Can you work these out from the model? Positions are in its coordinate system, mm. A direction names the side the tool comes from. Give positions to 0.01 mm unless a question says otherwise; leave off trailing zeros. Loops run counter-clockwise (first coordinate to the right, second up) from the corner with the lowest first, then second, coordinate; pieces in that order, holes last. Notation, with made-up numbers: (2.5, 20.5) -> (54.5, 20.5) arc R9 ccw to (54.5, 24.5) -> close; hole circle Ø1 at (-33.75, 61.5). An arc over 180 degrees is marked (long way). Return JSON: item names as keys, results as strings. Group by question number.
Q1. Suppose I cut it at C-C, the plane x = -27.75. Please give me the cut outline in (y, z), and give its area (3 significant figures).
Q2. Which directions (+Z, -Z, +X, -X, +Y, -Y) give clear straight access to the entire face, cutting with the end or side of a thin tool? Please do faces 4 (the flat face through (-15, 0, -15)), 5 (the flat face through (-3.5, 1, -21)), 6 (the flat face through (-26.5, 1, -3)).
Q3. Suppose I cut it at A-A, the plane y = 1.05. Please give me the cut outline in (x, z).
Q4. Suppose I cut it at B-B, the plane z = -24.5. Please give me the cut outline in (x, y), and give its area (3 significant figures).
Q5. Will this pin go through, and if not, where does the flat tip stop? pin 1 (12 mm diameter, centred on x = -20, z = -11, fed in from -Y).
Q6. I need wall thicknesses on line 1 along X through (y, z) = (1.3, -20.5); line 2 along Z through (x, y) = (-2.25, 0.75); line 3 along X through (y, z) = (1.2, -11). Which ranges of each line are inside material? Lowest first, please. Write a range as [from, to].
Q7. Thinking about a two-plate mould opening in X: for faces 1 (the flat face through (-26.5, 1, -21)), 2 (the flat face through (-3.5, 1, -3)), 3 (the flat face through (-15, 1.5, -15)), which applies, pulls with the +X half, pulls with the -X half, needs draft (parallel to the pull), parting line crosses it, or undercut?
Autodesk Inventor part; units mm, degrees
ref_plane "YZ Plane" through (0, 0, 0) normal (1, 0, 0) x (0, 1, 0)
ref_plane "XZ Plane" through (0, 0, 0) normal (0, 1, 0) x (-1, 0, 0)
ref_plane "XY Plane" through (0, 0, 0) normal (0, 0, 1) x (1, 0, 0)
sketch "スケッチ1" plane through (0, 0, 0) normal (0, 1, 0) x (-1, 0, 0)
  line L0 (0, 0) -> (30, 0)
  line L1 (30, 0) -> (30, -30)
  line L2 (30, -30) -> (0, -30)
  line L3 (0, -30) -> (0, 0)
  circle A0 centre (26.5, -9) radius 3.5
  circle A1 centre (3.5, -9) radius 3.5
  line L4 (26.5, 0) -> (26.5, -30)
  line L5 (3.5, -30) -> (3.5, 0)
  point P0 (26.5, -12.5)
  point P1 (26.5, -5.5)
  point P2 (3.5, -5.5)
  point P3 (3.5, -12.5)
  dimension "d0" = 30
  dimension "d1" = 30
  dimension "d2" = 7
  dimension "d3" = 7
  dimension "d4" = 9
extrude "押し出し1" add sketch "スケッチ1" along normal blind 1.5 contours L0 L4 A0 L2 L5 A1 | A1 L5 | A1 L5 | L4 A0 | A0 L4
properties part number "type_A"
Ans:
{
 "1": {"outline": "(0, -12.27) -> (1.5, -12.27) -> (1.5, -5.73) -> (0, -5.73) -> close", "area": "9.81 mm^2"},
 "2": {"face 4": "+Z, -Z, +X, -X, -Y", "face 5": "-Z, +X, +Y, -Y", "face 6": "+Z, -X, +Y, -Y"},
 "3": {"outline": "(-26.5, -30) -> (-3.5, -30) -> (-3.5, -12.5) arc R3.5 ccw to (-3.5, -5.5) -> (-3.5, 0) -> (-26.5, 0) -> (-26.5, -5.5) arc R3.5 ccw to (-26.5, -12.5) -> close"},
 "4": {"outline": "(-26.5, 0) -> (-3.5, 0) -> (-3.5, 1.5) -> (-26.5, 1.5) -> close", "area": "34.5 mm^2"},
 "5": {"pin 1": "stops at y = 0"},
 "6": {"line 1": "x = [-26.5, -3.5]", "line 2": "z = [-12.27, -5.73]", "line 3": "x = [-29.37, -0.63]"},
 "7": {"face 1": "pulls with the -X half", "face 2": "pulls with the +X half", "face 3": "needs draft"}
}
